Geometry: final body of the model. Coordinates: model frame, mm. Face numbers are marked on the shaded views. A direction names the side the tool comes from. Coordinates: 2 decimals unless noted, no trailing zeros. Loops run counter-clockwise (first coordinate to the right, second up) from the corner with the lowest first, then second, coordinate; pieces in that order, holes last. Notation, with made-up numbers: (0.25, -3) - (26.25, -3) arc R15 ccw to (26.25, 20) - close; hole circle Ø2 at (-30.75, -6). An arc over 180 degrees is marked (long way). Return JSON: item names as keys, results as strings.
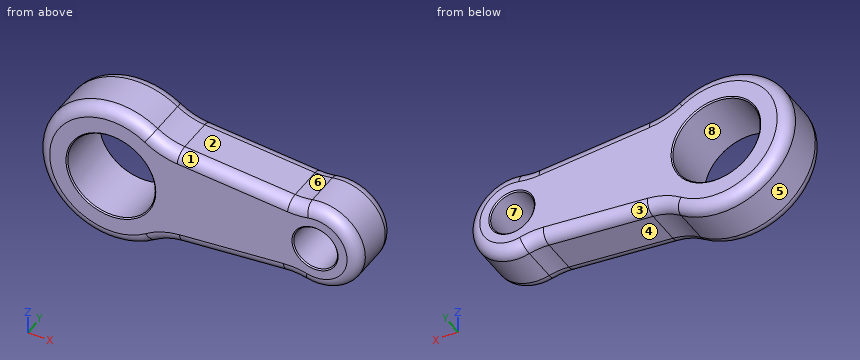
from build123d import *

# Parameters (mm, degrees)
F0_R     = 19.05
F0_R_2   = 9.525
F1_DEPTH = 12.7
F2_R     = 5.08
F3_SIZE  = 0.508


with BuildPart() as f1:
    # F0 (on Front) → F1 (new body, symmetric)
    with BuildSketch(Plane.XZ):
        with BuildLine():
            ThreePointArc((29.306325, 22.368523), (23.151754, 23.689977), (17.511156, 26.484371))
            ThreePointArc((17.511156, 26.484371), (-31.748308, -0.327731), (18.054151, -26.117238))
            ThreePointArc((18.054151, -26.117238), (23.882044, -23.116795), (30.283716, -21.707683))
            Line((30.283716, -21.707683), (75.603099, -17.742751))
            ThreePointArc((75.603099, -17.742751), (79.906584, -17.732206), (84.150081, -18.448327))
            ThreePointArc((84.150081, -18.448327), (107.945967, -0.391982), (84.913145, 18.628137))
            ThreePointArc((84.913145, 18.628137), (81.165755, 18.114123), (77.383583, 18.162308))
            Line((77.383583, 18.162308), (29.306325, 22.368523))
        make_face()
        Circle(F0_R, mode=Mode.SUBTRACT)
        with Locations((88.9, 0)):
            Circle(F0_R_2, mode=Mode.SUBTRACT)
    extrude(amount=F1_DEPTH, both=True)

    # F2
    f2_edges = [f1.edges().sort_by_distance(p)[0] for p in [
        (-31.748308, -12.7, -0.327731),
        (-31.748308, 12.7, -0.327731),
    ]]
    fillet(f2_edges, radius=F2_R)

    # F3
    f3_edges = [f1.edges().sort_by_distance(p)[0] for p in [
        (-19.05, -12.7, 0),
        (79.375, -12.7, 0),
        (-19.05, 12.7, 0),
        (79.375, 12.7, 0),
    ]]
    chamfer(f3_edges, length=F3_SIZE)


solid = f1.part
Item 1: Section query B-B, the plane z = 0. Count the separate pieces of the cut face and the enclosed holes in it, and give its area (3 significant figures).
Worked out:
{"separate pieces": "3", "enclosed holes": "0", "area": "2,070 mm^2"}
Item 2: Section query C-C, the plane y = -9.25. Return loops of the section in (x, z) (3 decimals).
Worked out:
{"outline": "(17.363, 26.26) arc R31.481 ccw (long way) to (17.901, -25.896) arc R25.669 cw to (30.26, -21.44) - (75.58, -17.475) arc R25.669 cw to (84.217, -18.188) arc R18.781 ccw (long way) to (84.969, 18.365) arc R25.669 cw to (77.36, 17.895) - (29.283, 22.101) arc R25.669 cw to start; hole circle Ø38.1 at (0, 0); hole circle Ø19.05 at (88.9, 0)"}
Item 3: Mould query, pull axis Z, two halves, no side actions, for the marked faces 5, 6, 7 and 8. Classes: +Z half, -Z half, draft (parallel to the pull), parting line (faces both ways), or undercut.
Worked out:
{"face 5": "parting line", "face 6": "+Z half", "face 7": "undercut", "face 8": "undercut"}
Item 4: First-contact query: pin 1 Ø8 at (y, z) = (4, -8.5) entering from +X; pin 2 Ø2 at (x, y) = (41.5, 9.5) entering from -Z; pin 3 Ø8 at (y, z) = (3, -14.5) entering from -X. Flat tips, straight axial feed; report the tip coordinate or a pass-through.
Worked out:
{"pin 1": "x = 107.41", "pin 2": "z = -20.67", "pin 3": "x = -29.96"}
Item 5: Ray query, probe 1 along Z at (x, y) = (0, -1.75); probe 2 along X at (y, z) = (-6, 6); probe 3 along Z at (x, y) = (88.9, -6) (3 decimals). Return the intervals inside material, ascending. Write a range as from..to.
Worked out:
{"probe 1": "-31.75..-19.05, 19.05..31.75", "probe 2": "-31.18..-18.08, 18.08..81.5, 96.3..106.98", "probe 3": "-19.05..-9.525, 9.525..19.05"}
Item 6: Reachability of the marked faces 1, 2, 3 and 4 from +Z, -Z, +X, -X, +Y, -Y: full face, straight path, thin tool, end or side. Return the list, or none.
Worked out:
{"face 1": "+Z, -Y", "face 2": "+Z, +Y, -Y", "face 3": "-Z, +Y", "face 4": "-Z, +Y, -Y"}
Item 7: Section query A-A, the plane y = 6.25. Return loops of the section in (x, z) (3 decimals).
Worked out:
{"outline": "(17.511, 26.484) arc R31.75 ccw (long way) to (18.054, -26.117) arc R25.4 cw to (30.284, -21.708) - (75.603, -17.743) arc R25.4 cw to (84.15, -18.448) arc R19.05 ccw (long way) to (84.913, 18.628) arc R25.4 cw to (77.384, 18.162) - (29.306, 22.369) arc R25.4 cw to start; hole circle Ø38.1 at (0, 0); hole circle Ø19.05 at (88.9, 0)"}
